Source: CAD feature listing. Evaluate the final solid. Frame: model axes, mm. Face numbers are marked on the shaded views. A direction names the side the tool comes from. Give positions to 0.01 mm unless a question says otherwise; leave off trailing zeros. Loops run counter-clockwise (first coordinate to the right, second up) from the corner with the lowest first, then second, coordinate; pieces in that order, holes last.
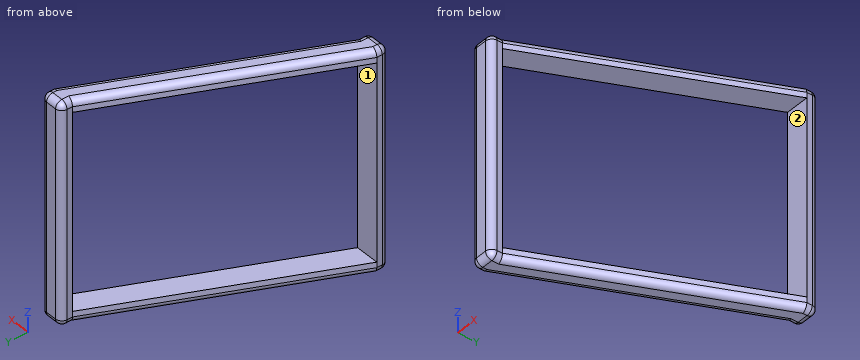
from build123d import *

# Parameters (mm, degrees)
PAD_DEPTH    = 1.5
SKETCH001_W  = 3
SKETCH001_H  = 1.5
PAD001_DEPTH = 25
PAD002_DEPTH = 1.5
FILLET_R     = 0.8


with BuildPart() as part:
    # Sketch → Pad (new body)
    with BuildSketch(Plane.XY):
        Polygon((0, 0), (0, 1.5), (-3, 1.5), (-3, 0), (-16, -28.25), (-16, -29.75), (-13, -29.75), (-13, -28.25), align=None)
    extrude(amount=PAD_DEPTH)

    # Sketch001 (on Face10 of Pad) → Pad001 (join)
    with BuildSketch(Plane.XY.offset(1.5)):
        with Locations((-1.5, 0.75)):
            Rectangle(SKETCH001_W, SKETCH001_H)
        with Locations((-14.5, -29)):
            Rectangle(SKETCH001_W, SKETCH001_H)
    extrude(amount=PAD001_DEPTH)

    # Sketch002 (on Face16 of Pad001) → Pad002 (join)
    with BuildSketch(Plane.XY.offset(26.5)):
        Polygon((-16, -28.25), (-3, 0), (-3, 1.5), (0, 1.5), (0, 0), (-13, -28.25), (-13, -29.75), (-16, -29.75), align=None)
    extrude(amount=PAD002_DEPTH)

    # Fillet
    fillet_edges = [part.edges().sort_by_distance(p)[0] for p in [
        (-16, -29.75, 14),
        (-13, -29.75, 14),
        (-14.5, -29.75, 0),
        (-14.5, -29.75, 28),
        (0, 1.5, 14),
        (-1.5, 1.5, 28),
        (-3, 1.5, 14),
        (-1.5, 1.5, 0),
        (0, 0.75, 0),
        (-6.5, -14.125, 0),
        (-13, -29, 0),
        (-3, 0.75, 0),
        (-9.5, -14.125, 0),
        (-16, -29, 0),
        (0, 0.75, 28),
        (-6.5, -14.125, 28),
        (-13, -29, 28),
        (-3, 0.75, 28),
        (-9.5, -14.125, 28),
        (-16, -29, 28),
    ]]
    fillet(fillet_edges, radius=FILLET_R)


solid = part.part
1) Cut plane A-A (z = 16.25). Return loops of the section in (x, y), and give its area (3 significant figures).
Checks:
outline: (-16, -28.95) arc R0.8 ccw to (-15.2, -29.75) - (-13.8, -29.75) arc R0.8 ccw to (-13, -28.95) - (-13, -28.25) - (-16, -28.25) - close; (-3, 0) - (0, 0) - (0, 0.7) arc R0.8 ccw to (-0.8, 1.5) - (-2.2, 1.5) arc R0.8 ccw to (-3, 0.7) - close
area: 8.45 mm2
2) Reachability of the marked faces 1 and 2 from +Z, -Z, +X, -X, +Y, -Y: full face, straight path, thin tool, end or side. Return the list, or none.
Checks:
face 1: +X, -X, +Y
face 2: +X, -X, -Y
3) Ray query, probe 1 along Y at (x, z) = (-14.5, 4.5); probe 2 along Y at (x, z) = (-2, 15); probe 3 along Z at (x, y) = (-10.75, -17). Return the intervals inside material, ascending.
Checks:
probe 1: y = -29.75 to -28.25
probe 2: y = 0 to 1.5
probe 3: z = 0.48 to 1.5, 26.5 to 27.52
4) Contact query for flat-ended pins moving along their axis: P1, Ø6, axis at x = -1.5, z = 18, coming from the -Y side; P2, Ø0.8, axis at y = -28.5, z = 15.5, coming from the +X side; P3, Ø0.6, axis at y = 0.5, z = 13, coming from the -X side; P4, Ø8, axis at x = -11.5, y = -24.5, coming from the -Z side. Output: stop coordinate, or through.
Checks:
P1: stops at y = 0
P2: stops at x = -13
P3: stops at x = -3
P4: stops at z = 0
